from build123d import *

# Parameters (mm, degrees)
SKETCH1_W               = 1.85
SKETCH1_H               = 47
CUT_EXTRUDE1_DEPTH      = 25.984995497
CUT_EXTRUDE1_DEPTH_BACK = 25.984995497
SKETCH2_R               = 0.75
FILLET1_R               = 0.5


with BuildPart() as part:
    # Sketch1 → Revolve1 (revolve)
    with BuildSketch(Plane(origin=(0, 0, 0), x_dir=(0, 0, -1), z_dir=(1, 0, 0)), mode=Mode.PRIVATE) as revolve1_sk:
        with Locations((5.075, 0)):
            Rectangle(SKETCH1_W, SKETCH1_H)
    revolve(revolve1_sk.sketch.rotate(Axis((0, 43.756475867, 0), (0, -1, 0)), 180), axis=Axis((0, 43.756475867, 0), (0, -1, 0)))

    # Sketch2 → Cut-Extrude1 (cut, two sides: drawn at the far end of the back side and taken through both)
    with BuildSketch(Plane(origin=(0, 0, 0), x_dir=(0, 0, -1), z_dir=(1, 0, 0)).offset(-CUT_EXTRUDE1_DEPTH_BACK)):
        with Locations((0, 18.5)):
            Circle(SKETCH2_R)
        with Locations((0, -18.5)):
            Circle(SKETCH2_R)
    extrude(amount=CUT_EXTRUDE1_DEPTH + CUT_EXTRUDE1_DEPTH_BACK, mode=Mode.SUBTRACT)

    # Fillet1
    fillet1_edges = [part.edges().sort_by_distance(p)[0] for p in [
        (0, -23.5, -6),
        (0, 23.5, -6),
    ]]
    fillet(fillet1_edges, radius=FILLET1_R)


solid = part.part
The model under review builds one solid part; all positions refer to its coordinate system, in mm. Coordinates: 2 decimals unless noted, no trailing zeros. Write each loop counter-clockwise with the first axis right and the second up, starting at its lowest first coordinate (ties: lowest second). Pieces come first, ordered by that corner, then holes. Notation, with made-up numbers: (30.25, 51) - (35.25, 51) arc R20 cw to (35.25, 68) - close; hole circle Ø1 at (-31, 72.25). An arc over 180 degrees is marked (long way). Answer as a JSON object with one key per item and string values. Group by question number.
1. Add section D-D (y = -3.5). Give the boundary of the cut face in (x, z), plus the area to 3 significant figures.
2. To check wall thickness, follow probe 1 along Y at (x, z) = (-5.25, 0); probe 2 along X at (y, z) = (13, 0); probe 3 along Z at (x, y) = (3, 6.5). State the ranges of each line that lie inside material, in increasing order.
3. Add section B-B (x = 0). Give the boundary of the cut face in (y, z).
4. Add section A-A (z = 0). Give the boundary of the cut face in (x, y), plus the area to 3 significant figures.
5. Mouldability with a two-part tool opening along Y and no side actions: class faces 1 (the face through (5.027, 17.768, 0.163)), 2 (the face through (-4, -23.5, 2)), 3 (the face through (-5.054, 17.768, 0.163)), 4 (the face through (-4, 23.5, 2)) as pulls with the +Y half, pulls with the -Y half, needs draft (parallel to the pull), parting line crosses it, or undercut.
6. Clearance check with flat-ended pins moving along their axes: pin 1 Ø5 at (x, y) = (-4.5, 10.5) entering from -Z; pin 2 Ø1.2 at (y, z) = (-18.5, 0) entering from -X; pin 3 Ø6 at (y, z) = (0, -3) entering from +X; pin 4 Ø2 at (x, y) = (-2.5, 2) entering from +Z. State where each tip first meets the part, or that it passes through.
7. Add section C-C (y = 18.5). Give the boundary of the cut face in (x, z), plus the area to 3 significant figures.
Findings:
{
 "1": {"outline": "circle Ø12 at (0, 0); hole circle Ø8.3 at (0, 0)", "area": "59.0 mm²"},
 "2": {"probe 1": "-23.5 to -19.25, -17.75 to 17.75, 19.25 to 23.5", "probe 2": "-6 to -4.15, 4.15 to 6", "probe 3": "-5.2 to -2.87, 2.87 to 5.2"},
 "3": {"outline": "(-23.5, -5.5) arc R0.5 ccw to (-23, -6) - (23, -6) arc R0.5 ccw to (23.5, -5.5) - (23.5, -4.15) - (-23.5, -4.15) - close; (-23.5, 4.15) - (23.5, 4.15) - (23.5, 5.5) arc R0.5 ccw to (23, 6) - (-23, 6) arc R0.5 ccw to (-23.5, 5.5) - close"},
 "4": {"outline": "(-6, -23) arc R0.5 ccw to (-5.5, -23.5) - (-4.15, -23.5) - (-4.15, -19.25) - (-6, -19.25) - close; (-6, -17.75) - (-4.15, -17.75) - (-4.15, 17.75) - (-6, 17.75) - close; (-6, 19.25) - (-4.15, 19.25) - (-4.15, 23.5) - (-5.5, 23.5) arc R0.5 ccw to (-6, 23) - close; (4.15, -23.5) - (5.5, -23.5) arc R0.5 ccw to (6, -23) - (6, -19.25) - (4.15, -19.25) - close; (4.15, -17.75) - (6, -17.75) - (6, 17.75) - (4.15, 17.75) - close; (4.15, 19.25) - (6, 19.25) - (6, 23) arc R0.5 ccw to (5.5, 23.5) - (4.15, 23.5) - close", "area": "163 mm²"},
 "5": {"face 1": "undercut", "face 2": "pulls with the -Y half", "face 3": "undercut", "face 4": "pulls with the +Y half"},
 "6": {"pin 1": "z = -5.66", "pin 2": "through", "pin 3": "x = 6", "pin 4": "z = 5.81"},
 "7": {"outline": "(-5.95, -0.75) arc R6 ccw to (5.95, -0.75) - (4.08, -0.75) arc R4.15 cw to (-4.08, -0.75) - close; (-5.95, 0.75) - (-4.08, 0.75) arc R4.15 cw to (4.08, 0.75) - (5.95, 0.75) arc R6 ccw to start", "area": "53.4 mm²"}
}
